Read the model definition and answer for the solid it produces. Units are mm, in the model's axes. A direction names the side the tool comes from. Coordinates: 2 decimals unless noted, no trailing zeros. Write each loop counter-clockwise with the first axis right and the second up, starting at its lowest first coordinate (ties: lowest second). Pieces come first, ordered by that corner, then holes.
(1) Which of the six approach directions +Z, -Z, +X, -X, +Y, -Y give full straight-line access (tool end or side, diameter ignored) to faces 4 (the flat face through (-6.35, 3, 19)), 5 (the flat face through (0, 3, -6.35)), 6 (the flat face through (19.05, 3, -19)), 7 (the cylindrical face through (34.823, 4.002, -0.688)), 8 (the cylindrical face through (19.774, 3.131, 7.114))?
(2) Find the intervals of material crossed by probe 1 along X at (y, z) = (6.25, -12); probe 2 along X at (y, z) = (4.6, 0); probe 3 along Z at (x, y) = (-12.7, 3.75) (3 decimals), in increasing order.
(3) Given pin 1 (3 mm diameter, centred on x = 47, y = 3.5, fed in from -Z); pin 2 (5 mm diameter, centred on x = -60.325, z = 0, fed in from +Y); pin 3 (10 mm diameter, centred on x = 37.92, z = 0, fed in from -Y), each flat-ended and moving along its own axis, determine where each tip first touches the part or whether it passes through.
(4) Section C-C on y = 3.75 is taken. State how many separate pieces and enclosed holes the cut face has, then the cut area to 3 significant figures.
(5) Section A-A on z = -22 is taken. Write down the section's boundary in (x, y), then the cut area to 3 significant figures.
(6) Section B-B on x = 49.5 is taken. Write down the section's boundary in (y, z), then the cut area to 3 significant figures.
(7) The mould has two halves that part along X. Classify faces 1 (the flat face through (-19.05, 3, 19)), 2 (the cylindrical face through (17.141, 3.131, 33.114)), 3 (the cylindrical face through (8.161, 3.131, 33.016)): +X half, -X half, draft (parallel to the pull), parting line (faces both ways), or undercut.
from build123d import *

# Parameters (mm, degrees)
SKETCH1_W                 = 139.7
SKETCH1_H                 = 12.7
BOSS_EXTRUDE1_DEPTH       = 6.35
SKETCH2_R                 = 3.175
CUT_EXTRUDE2_DEPTH        = 4.7625
SKETCH3_R                 = 3.175
CUT_EXTRUDE3_DEPTH        = 4.7625
FILLET1_R                 = 6.35
F_6_CLEARANCE_HOLE1_D     = 3.7973
F_6_CLEARANCE_HOLE1_DEPTH = 25.4
F_6_CLEARANCE_HOLE1_TIP   = 1.140824014
F_6_CLEARANCE_HOLE2_D     = 3.7973
F_6_CLEARANCE_HOLE2_DEPTH = 25.4
F_6_CLEARANCE_HOLE2_TIP   = 1.140824014
SKETCH8_W                 = 12.7
SKETCH8_H                 = 69.85
BOSS_EXTRUDE2_DEPTH       = 6.35
F_6_CLEARANCE_HOLE3_D     = 3.7973
F_6_CLEARANCE_HOLE3_DEPTH = 25.4
F_6_CLEARANCE_HOLE3_TIP   = 1.140824014
FILLET2_R                 = 2.54
FILLET3_R                 = 6.35


with BuildPart() as part:
    # Sketch1 → Boss-Extrude1 (new body)
    with BuildSketch(Plane(origin=(0, 0, 0), x_dir=(1, 0, 0), z_dir=(0, 1, 0))):
        Rectangle(SKETCH1_W, SKETCH1_H)
    extrude(amount=BOSS_EXTRUDE1_DEPTH)

    # Sketch2 → Cut-Extrude2 (cut)
    with BuildSketch(Plane(origin=(0, 6.35, 0), x_dir=(1, 0, 0), z_dir=(0, 1, 0))):
        with Locations(Location((-60.325, 0, 0), (0, 0, 270))):
            Circle(SKETCH2_R)
        with Locations(Location((37.9222, 0, 0), (0, 0, 270))):
            Circle(SKETCH2_R)
        with Locations(Location((60.52312, 0, 0), (0, 0, 270))):
            Circle(SKETCH2_R)
    extrude(amount=-CUT_EXTRUDE2_DEPTH, mode=Mode.SUBTRACT)

    # Sketch3 → Cut-Extrude3 (cut)
    with BuildSketch(Plane.XZ):
        with Locations(Location((-12.7, 0, 0), (0, 0, 270))):
            Circle(SKETCH3_R)
        with Locations(Location((12.7, 0, 0), (0, 0, 270))):
            Circle(SKETCH3_R)
    extrude(amount=-CUT_EXTRUDE3_DEPTH, mode=Mode.SUBTRACT)

    # Fillet1
    fillet1_edges = [part.edges().sort_by_distance(p)[0] for p in [
        (69.85, 3.175, 6.35),
        (69.85, 3.175, -6.35),
        (-69.85, 3.175, 6.35),
        (-69.85, 3.175, -6.35),
    ]]
    fillet(fillet1_edges, radius=FILLET1_R - 0.0001)  # a hair under: the kernel refuses the full size

    # #6 Clearance Hole1
    with Locations(Plane(origin=(0, 1.5875, 0), x_dir=(-1, 0, 0), z_dir=(0, 1, 0))):
        with Locations((-60.52312, 0), (-37.9222, 0), (60.325, 0)):
            Hole(F_6_CLEARANCE_HOLE1_D / 2, depth=F_6_CLEARANCE_HOLE1_DEPTH)
            with Locations((0, 0, -(F_6_CLEARANCE_HOLE1_DEPTH + F_6_CLEARANCE_HOLE1_TIP / 2))):  # 118° drill point
                Cone(0, F_6_CLEARANCE_HOLE1_D / 2, F_6_CLEARANCE_HOLE1_TIP, mode=Mode.SUBTRACT)

    # #6 Clearance Hole2
    with Locations(Plane.XZ.offset(-4.7625)):
        with Locations((-12.7, 0), (12.7, 0)):
            Hole(F_6_CLEARANCE_HOLE2_D / 2, depth=F_6_CLEARANCE_HOLE2_DEPTH)
            with Locations((0, 0, -(F_6_CLEARANCE_HOLE2_DEPTH + F_6_CLEARANCE_HOLE2_TIP / 2))):  # 118° drill point
                Cone(0, F_6_CLEARANCE_HOLE2_D / 2, F_6_CLEARANCE_HOLE2_TIP, mode=Mode.SUBTRACT)

    # Sketch8 → Boss-Extrude2 (add)
    with BuildSketch(Plane(origin=(0, 6.35, 0), x_dir=(1, 0, 0), z_dir=(0, 1, 0))):
        with Locations((-12.7, 0)):
            Rectangle(SKETCH8_W, SKETCH8_H)
        with Locations((12.7, 0)):
            Rectangle(SKETCH8_W, SKETCH8_H)
    extrude(amount=-BOSS_EXTRUDE2_DEPTH)

    # #6 Clearance Hole3
    with Locations(Plane(origin=(0, 6.35, 0), x_dir=(-1, 0, 0), z_dir=(0, 1, 0))):
        with Locations((12.7, -28.575), (12.7, 28.575), (-12.7, 28.575), (-12.7, -28.575)):
            Hole(F_6_CLEARANCE_HOLE3_D / 2, depth=F_6_CLEARANCE_HOLE3_DEPTH)
            with Locations((0, 0, -(F_6_CLEARANCE_HOLE3_DEPTH + F_6_CLEARANCE_HOLE3_TIP / 2))):  # 118° drill point
                Cone(0, F_6_CLEARANCE_HOLE3_D / 2, F_6_CLEARANCE_HOLE3_TIP, mode=Mode.SUBTRACT)

    # Fillet2
    fillet2_edges = [part.edges().sort_by_distance(p)[0] for p in [
        (6.35, 3.175, 6.35),
        (6.35, 3.175, -6.35),
        (19.05, 3.175, 6.35),
        (19.05, 3.175, -6.35),
        (-19.05, 3.175, 6.35),
        (-19.05, 3.175, -6.35),
        (-6.35, 3.175, 6.35),
        (-6.35, 3.175, -6.35),
    ]]
    fillet(fillet2_edges, radius=FILLET2_R)

    # Fillet3
    fillet3_edges = [part.edges().sort_by_distance(p)[0] for p in [
        (19.05, 3.175, -34.925),
        (6.35, 3.175, -34.925),
        (-6.35, 3.175, -34.925),
        (-19.05, 3.175, -34.925),
        (-19.05, 3.175, 34.925),
        (-6.35, 3.175, 34.925),
        (6.35, 3.175, 34.925),
        (19.05, 3.175, 34.925),
    ]]
    fillet(fillet3_edges, radius=FILLET3_R - 0.0001)  # a hair under: the kernel refuses the full size


solid = part.part
Response:
1. face 4: +Z, +Y, -Y
1. face 5: -Z, +Y, -Y
1. face 6: -Z, +X, +Y, -Y
1. face 7: +Y
1. face 8: +Z, +X, +Y, -Y
2. probe 1: x = -19.05 to -6.35, 6.35 to 19.05
2. probe 2: x = -69.85 to -63.5, -57.15 to 34.75, 41.1 to 57.35, 63.7 to 69.85
2. probe 3: z = -34.925 to -30.474, -26.676 to 26.676, 30.474 to 34.925
3. pin 1: stops at z = -6.35
3. pin 2: stops at y = 1.59
3. pin 3: stops at y = 0
4. separate pieces: 1
4. enclosed holes: 7
4. area: 2,990 mm2
5. outline: (-19.05, 0) - (-6.35, 0) - (-6.35, 6.35) - (-19.05, 6.35) - close; (6.35, 0) - (19.05, 0) - (19.05, 6.35) - (6.35, 6.35) - close
5. area: 161 mm2
6. outline: (0, -6.35) - (6.35, -6.35) - (6.35, 6.35) - (0, 6.35) - close
6. area: 80.6 mm2
7. face 1: -X half
7. face 2: +X half
7. face 3: undercut
